Work out the finished part from the listing and answer in its coordinate system (mm). Face numbers are marked on the shaded views. A direction names the side the tool comes from. Give positions to 0.01 mm unless a question says otherwise; leave off trailing zeros. Order: outer loops, then holes, each group sorted by start corner. A loop starts at its lowest first (then second) coordinate and runs counter-clockwise, first axis right, second up. Notation, with made-up numbers: M 53,-22.75 L 70,-22.75 A8 cw 70,-15.75 Z; hole C 25.25,-36.5 d4. An arc over 180 degrees is marked long. One line per item, written item: value.
from build123d import *

# Parameters (mm, degrees)
SKETCH_1_R          = 1.5
EXTRUDE_1_DEPTH     = 5
SKETCH_2_R          = 2.85
EXTRUDE_2_DEPTH     = 3
CUT_EXTRUDE_1_DEPTH = 1
CHAMFER_1_SIZE      = 0.2


with BuildPart() as part:
    # 草图1 → 凸台-拉伸1 (new body)
    with BuildSketch(Plane(origin=(0, 0, 0), x_dir=(1, 0, 0), z_dir=(0, 1, 0))):
        with Locations(Location((0, 0, 0), (0, 0, 270))):
            Circle(SKETCH_1_R)
    extrude(amount=EXTRUDE_1_DEPTH)

    # 草图2 → 凸台-拉伸2 (add)
    with BuildSketch(Plane.XZ):
        with Locations(Location((0, 0, 0), (0, 0, 270))):
            Circle(SKETCH_2_R)
    extrude(amount=EXTRUDE_2_DEPTH)

    # 草图3 → 切除-拉伸1 (cut)
    with BuildSketch(Plane.XZ.offset(3)):
        Polygon((1.443375673, 0), (0.721687836, 1.25), (-0.721687836, 1.25), (-1.443375673, 0), (-0.721687836, -1.25), (0.721687836, -1.25), align=None)
    extrude(amount=-CUT_EXTRUDE_1_DEPTH, mode=Mode.SUBTRACT)

    # 倒角1
    chamfer_1_edges = [part.edges().sort_by_distance(p)[0] for p in [
        (0, -3, 2.85),
    ]]
    chamfer(chamfer_1_edges, length=CHAMFER_1_SIZE)


solid = part.part
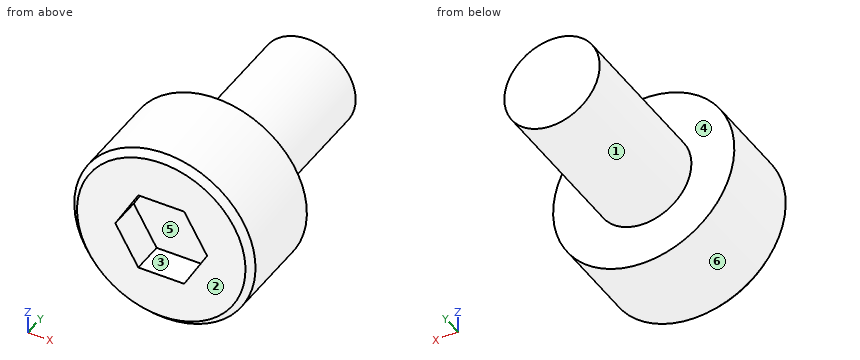
(1) Given P1, Ø2, axis at y = -2, z = 1.5, coming from the +X side; P2, Ø1, axis at y = 1.5, z = 1, coming from the -X side, each flat-ended and moving along its own axis, determine where each tip first touches the part or whether it passes through.
Findings:
P1: stops at x = 2.81
P2: stops at x = -1.41
(2) Determine the mould class of the marked faces 1, 2 and 3 for opening direction Z: pulls with the +Z half, pulls with the -Z half, needs draft (parallel to the pull), parting line crosses it, or undercut.
Findings:
face 1: parting line crosses it
face 2: needs draft
face 3: undercut
(3) Section A-A, the plane x = 0 is taken. Give the vertices of the cut face in (y, z).
Findings:
outline: M -3,-2.65 L -2.8,-2.85 L 0,-2.85 L 0,-1.5 L 5,-1.5 L 5,1.5 L 0,1.5 L 0,2.85 L -2.8,2.85 L -3,2.65 L -3,1.25 L -2,1.25 L -2,-1.25 L -3,-1.25 Z
(4) Section B-B, the plane y = 2.5 is taken. Give the vertices of the cut face in (x, z), then the cut area to 3 significant figures.
Findings:
outline: C 0,0 d3
area: 7.07 mm^2
(5) Which of the six approach directions +Z, -Z, +X, -X, +Y, -Y give full straight-line access (tool end or side, diameter ignored) to the marked faces 4, 5 and 6?
Findings:
face 4: +Y
face 5: -Y
face 6: +Y, -Y
(6) Section C-C, the plane y = -0.5 is taken. Give the vertices of the cut face in (x, z).
Findings:
outline: C 0,0 d5.7
(7) Find the intervals of material crossed by probe 1 along Y at (x, z) = (1.9, 0.15); probe 2 along Z at (x, y) = (-0.4, -2.5); probe 3 along Y at (x, z) = (-0.3, 0.5), in increasing order. Write a range as from..to.
Findings:
probe 1: y = -3..0
probe 2: z = -2.82..-1.25, 1.25..2.82
probe 3: y = -2..5
